Autodesk Inventor part; units mm, degrees
ref_plane "XZ Plane" through (0, 0, 0) normal (0, 1, 0) x (-1, 0, 0)
ref_plane "XY Plane" through (0, 0, 0) normal (0, 0, 1) x (1, 0, 0)
sketch "Skizze1" plane through (0, 0, 0) normal (0, 0, 1) x (1, 0, 0)
  line L0 (-4.75, 4.75) -> (4.75, 4.75)
  line L1 (4.75, 4.75) -> (4.75, -4.75)
  line L2 (4.75, -4.75) -> (-4.75, -4.75)
  line L3 (-4.75, -4.75) -> (-4.75, 4.75)
  line L4 (-4.75, 4.75) -> (4.75, -4.75) construction
  line L5 (4.75, 4.75) -> (-4.75, -4.75) construction
  point P0 (0, 0)
  dimension "d0" = 9.5
  dimension "d1" = 9.5
extrude "Extrusion1" add sketch "Skizze1" along normal blind 3.5
sketch "Skizze2" plane through (0, 0, 3.5) normal (0, 0, 1) x (1, 0, 0)
  circle A0 centre (0, 0) radius 8.5
  dimension "d4" = 17
extrude "Extrusion2" add sketch "Skizze2" along normal blind 3
sketch "Skizze3" plane through (0, 0, 6.5) normal (0, 0, 1) x (1, 0, 0)
  circle A0 centre (0, 0) radius 7.4
  circle A1 centre (0, 0) radius 8.5
  dimension "d7" = 14.8
  dimension "d19" = 1.1
extrude "Extrusion3" add sketch "Skizze3" along normal blind 130 contours A0
sketch "Skizze4" plane through (0, 0, 136.5) normal (0, 0, 1) x (1, 0, 0)
  line L0 (-4.75, -4.75) -> (4.75, -4.75)
  line L1 (-4.75, 4.75) -> (4.75, 4.75)
  line L2 (4.75, 4.75) -> (4.75, -4.75)
  line L3 (4.75, -4.75) -> (-4.75, -4.75)
  line L4 (-4.75, -4.75) -> (-4.75, 4.75)
  line L5 (-4.75, 4.75) -> (4.75, -4.75) construction
  line L6 (4.75, 4.75) -> (-4.75, -4.75) construction
  point P0 (0, 0)
  dimension "d10" = 9.5
extrude "Extrusion4" add sketch "Skizze4" along normal blind 6
sketch "Skizze5" plane through (0, 0, 142.5) normal (0, 0, 1) x (1, 0, 0)
  circle A0 centre (0, 0) radius 2.25
  dimension "d13" = 4.5
extrude "Extrusion5" cut sketch "Skizze5" against normal blind 5
sketch "Skizze6" plane through (0, 0, 0) normal (0, 0, -1) x (-1, 0, 0)
  circle A0 centre (0, 0) radius 2.25
  dimension "d16" = 4.5
extrude "Extrusion6" cut sketch "Skizze6" against normal blind 5
properties part number "_3D-Druck"
Build history of the part. All positions in model axes, mm. A direction names the side the tool comes from. Round coordinates to 2 decimals unless told otherwise and drop trailing zeros. Write each loop counter-clockwise with the first axis right and the second up, starting at its lowest first coordinate (ties: lowest second). Pieces come first, ordered by that corner, then holes. Notation, with made-up numbers: M 56,-2 L 98,-2 A20 cw 98,20 Z; hole C 44.5,75.5 d5. An arc over 180 degrees is marked long. Answer as a JSON object with one key per item and string values. Group by question number.
(1) Cut at A-A (x = 0). Give the cut face in (y, z), and give its area (3 significant figures).
(2) Drill centre lines: L1, parallel to Y at x = 0, z = 141; L2, parallel to Y at x = 0, z = 3.75; L3, parallel to Z at x = 2, y = -6.5. Where is each one in solid material? Low to high.
(3) Mould opens along Y. For faces 1 (the flat face through (0, -4.75, 2)), 2 (the flat face through (-3, 7, 6.5)), 3 (the cylindrical face through (-1.604, 7.224, 70.59)), 4 (the cylindrical face through (0.29, 2.23, 2.46)) say: pulls with the +Y half, pulls with the -Y half, needs draft (parallel to the pull), parting line crosses it, or undercut.
(4) Cut at C-C (z = 76). Give the cut face in (x, y).
(5) Flat gauge pins, fed straight in: pin 1 (1 mm diameter, centred on y = -1.5, z = 2, fed in from +X); pin 2 (1.3 mm diameter, centred on x = -1, y = 1, fed in from -Z); pin 3 (2 mm diameter, centred on x = -3, z = 112, fed in from -Y). Where does each tip first touch, or does it go through?
(6) Which spindle directions (+Z, -Z, +X, -X, +Y, -Y) get a long thin tool onto all of the face, cutting with end or side? Do faces 5 (the flat face through (0, 0, 5)), 6 (the flat face through (0, 0, 137.5)), 7 (the flat face through (0, -4.75, 139)). Say none if no direction does.
Responses:
{
 "1": {"outline": "M -8.5,3.5 L -4.75,3.5 L -4.75,0 L -2.25,0 L -2.25,5 L 2.25,5 L 2.25,0 L 4.75,0 L 4.75,3.5 L 8.5,3.5 L 8.5,6.5 L 7.4,6.5 L 7.4,136.5 L 4.75,136.5 L 4.75,142.5 L 2.25,142.5 L 2.25,137.5 L -2.25,137.5 L -2.25,142.5 L -4.75,142.5 L -4.75,136.5 L -7.4,136.5 L -7.4,6.5 L -8.5,6.5 Z", "area": "2,020 mm2"},
 "2": {"L1": "y = -4.75 to -2.25, 2.25 to 4.75", "L2": "y = -8.5 to -2.25, 2.25 to 8.5", "L3": "z = 3.5 to 136.5"},
 "3": {"face 1": "pulls with the -Y half", "face 2": "needs draft", "face 3": "parting line crosses it", "face 4": "undercut"},
 "4": {"outline": "C 0,0 d14.8"},
 "5": {"pin 1": "stops at x = 4.75", "pin 2": "stops at z = 5", "pin 3": "stops at y = -7.12"},
 "6": {"face 5": "-Z", "face 6": "+Z", "face 7": "+Z, +X, -X, -Y"}
}
